```python
from build123d import *

# Parameters (mm, degrees)
BOSS_EXTRUDE1_DEPTH = 35
CUT_EXTRUDE1_DEPTH  = 32
SKETCH5_W           = 4
SKETCH5_H           = 106
CUT_EXTRUDE2_DEPTH  = 32
SKETCH6_W           = 3
SKETCH6_H           = 106
CUT_EXTRUDE3_DEPTH  = 1.5
SKETCH7_W           = 3
SKETCH7_H           = 33.5
CUT_EXTRUDE4_DEPTH  = 1.5
CUT_EXTRUDE5_DEPTH  = 10
BOSS_EXTRUDE2_DEPTH = 33.5
BOSS_EXTRUDE3_DEPTH = 109


with BuildPart() as part:
    # PCB → Boss-Extrude1 (new body)
    with BuildSketch(Plane(origin=(0, 0, 0), x_dir=(1, 0, 0), z_dir=(0, 1, 0))):
        Polygon((68.5, -75.988917258), (118.036460317, -105.5), (135, -105.5), (136, -105.5), (136, 3.5), (135, 3.5), (-3.5, 3.5), (-3.5, -71), (68.5, -71), align=None)
    extrude(amount=BOSS_EXTRUDE1_DEPTH)

    # Sketch4 → Cut-Extrude1 (cut)
    with BuildSketch(Plane(origin=(0, 35, 0), x_dir=(1, 0, 0), z_dir=(0, 1, 0))):
        Polygon((133, 0.5), (-0.5, 0.5), (-0.5, -68), (71.5, -68), (71.5, -74.284131037), (118.862351474, -102.5), (133, -102.5), align=None)
    extrude(amount=-CUT_EXTRUDE1_DEPTH, mode=Mode.SUBTRACT)

    # Sketch5 → Cut-Extrude2 (cut)
    with BuildSketch(Plane(origin=(0, 35, 0), x_dir=(1, 0, 0), z_dir=(0, 1, 0))):
        with Locations((134, -49.5)):
            Rectangle(SKETCH5_W, SKETCH5_H)
    extrude(amount=-CUT_EXTRUDE2_DEPTH, mode=Mode.SUBTRACT)

    # Sketch6 → Cut-Extrude3 (cut)
    with BuildSketch(Plane(origin=(0, 3, 0), x_dir=(1, 0, 0), z_dir=(0, 1, 0))):
        with Locations((133.5, -49.5)):
            Rectangle(SKETCH6_W, SKETCH6_H)
    extrude(amount=-CUT_EXTRUDE3_DEPTH, mode=Mode.SUBTRACT)

    # Sketch7 → Cut-Extrude4 (cut)
    with BuildSketch(Plane(origin=(0, 0, 102.5), x_dir=(-1, 0, 0), z_dir=(0, 0, -1))):
        with Locations((-133.5, 18.25)):
            Rectangle(SKETCH7_W, SKETCH7_H)
    extrude(amount=-CUT_EXTRUDE4_DEPTH, mode=Mode.SUBTRACT)

    # Sketch10 → Cut-Extrude5 (cut)
    with BuildSketch(Plane(origin=(0, 35, 0), x_dir=(1, 0, 0), z_dir=(0, 1, 0))):
        Polygon((130.8, -105.5), (118.036460317, -105.5), (68.5, -75.988917258), (68.5, -71), (-3.5, -71), (-3.5, 3.5), (132, 3.5), (132, 1.7), (-1.7, 1.7), (-1.7, -69.2), (70.3, -69.2), (70.3, -74.966045525), (118.531995011, -103.7), (130.8, -103.7), align=None)
    extrude(amount=-CUT_EXTRUDE5_DEPTH, mode=Mode.SUBTRACT)

    # Sketch11 → Boss-Extrude2 (add)
    with BuildSketch(Plane(origin=(0, 1.5, 0), x_dir=(1, 0, 0), z_dir=(0, 1, 0))):
        Polygon((132, -104), (135, -102.5), (135, -104), align=None)
    extrude(amount=BOSS_EXTRUDE2_DEPTH)

    # Sketch13 → Boss-Extrude3 (add)
    with BuildSketch(Plane.XY.offset(105.5)):
        Polygon((132, 1.5), (135, 3), (135, 1.5), align=None)
    extrude(amount=-BOSS_EXTRUDE3_DEPTH)


solid = part.part
```
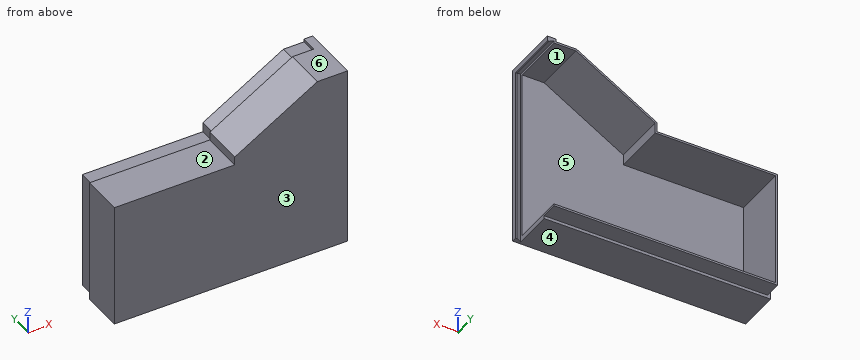
The model under review builds one solid part; all positions refer to its coordinate system, in mm. Face numbers are marked on the shaded views. A direction names the side the tool comes from. Round coordinates to 2 decimals unless told otherwise and drop trailing zeros. Write each loop counter-clockwise with the first axis right and the second up, starting at its lowest first coordinate (ties: lowest second). Pieces come first, ordered by that corner, then holes. Notation, with made-up numbers: M -1,88 L 30,88 A17 ccw 30,110 Z; hole C 75,44.5 d6. An arc over 180 degrees is marked long. Use CSV: the item, a comma, the result in double quotes. Start each with the question number.
(1) We need section C-C, the plane x = 59. State the section outline as (y, z) points.
(2) The part is to be moulded in two halves that separate along Z. For the marked faces 4, 5 and 6, say which applies: +Z half, -Z half, draft (parallel to the pull), parting line (faces both ways), or undercut.
(3) Tool access review of the marked faces 1, 2 and 3: name each direction out of +Z, -Z, +X, -X, +Y, -Y from which nothing blocks a thin tool from reaching the whole face with its end or side.
(4) Clearance check with flat-ended pins moving along their axes: P1, Ø5, axis at x = 126, y = 28.5, coming from the +Z side; P2, Ø7, axis at y = 13.5, z = 72, coming from the +X side; P3, Ø10, axis at y = 14.5, z = 45.5, coming from the +X side. State where each tip first meets the part, or that it passes through.
(5) We need section B-B, the plane z = 41. State the section outline as (x, y) points.
(6) For line 1 along Z through (x, y) = (31, 34.5); line 2 along Z through (x, y) = (42.5, 18); line 3 along Y through (x, z) = (127, 38), list the stretches that pass through material, from the lowest coordinate up.
(7) We need section A-A, the plane y = 30.5. State the section outline as (x, z) points, then the cut area to 3 significant figures.
(8) We need section D-D, the plane y = 6.5. State the section outline as (x, z) points, then the cut area to 3 significant figures.
Findings:
1,outline,"M 0,-3.5 L 25,-3.5 L 25,-1.7 L 35,-1.7 L 35,-0.5 L 3,-0.5 L 3,68 L 35,68 L 35,69.2 L 25,69.2 L 25,71 L 0,71 Z"
2,face 4,"-Z half"
2,face 5,"undercut"
2,face 6,"+Z half"
3,face 1,"+X, +Y"
3,face 2,"+Z, -X, +Y, -Y"
3,face 3,"+Z, -Z, +X, -X, -Y"
4,P1,"z = 103.7"
4,P2,"x = 73.54"
4,P3,"x = -0.5"
5,outline,"M -3.5,0 L 136,0 L 136,3 L 135,3 L 132,1.5 L 132,3 L -0.5,3 L -0.5,35 L -1.7,35 L -1.7,25 L -3.5,25 Z"
6,line 1,"-1.7 to -0.5, 68 to 69.2"
6,line 2,"-3.5 to -0.5, 68 to 71"
6,line 3,"0 to 3"
7,outline,"M -1.7,-1.7 L 132,-1.7 L 132,-0.5 L -0.5,-0.5 L -0.5,68 L 71.5,68 L 71.5,74.28 L 118.86,102.5 L 132,102.5 L 132,104 L 135,102.5 L 136,102.5 L 136,105.5 L 130.8,105.5 L 130.8,103.7 L 118.53,103.7 L 70.3,74.97 L 70.3,69.2 L -1.7,69.2 Z"
7,area,"432 mm^2"
8,outline,"M -3.5,-3.5 L 132,-3.5 L 132,-0.5 L -0.5,-0.5 L -0.5,68 L 71.5,68 L 71.5,74.28 L 118.86,102.5 L 132,102.5 L 132,104 L 135,102.5 L 136,102.5 L 136,105.5 L 118.04,105.5 L 68.5,75.99 L 68.5,71 L -3.5,71 Z"
8,area,"1,070 mm^2"
